CAD build for the part. Positions are in the model's coordinates, mm. Face numbers are marked on the shaded views. A direction names the side the tool comes from. Coordinates: 2 decimals unless noted, no trailing zeros. Loops run counter-clockwise (first coordinate to the right, second up) from the corner with the lowest first, then second, coordinate; pieces in that order, holes last.
1) Wall check: line 1 along Y through (x, z) = (-3.5, -20.15); line 2 along Z through (x, y) = (-1, -13.5); line 3 along Z through (x, y) = (19, -21). Give the ranges that are in metal, low to high.
2) Saw through at C-C, the plane z = -20.15. Write the cut outline in (x, y).
3) Which spindle directions (+Z, -Z, +X, -X, +Y, -Y) get a long thin tool onto all of the face, cutting with end or side? Do the marked faces 1, 2 and 3. Say none if no direction does.
4) Two-plate mould, pull along Z, no slides. Class the marked faces 4, 5 and 6: +Z half, -Z half, draft (parallel to the pull), parting line (faces both ways), or undercut.
5) Pin check, flat tips, straight feed: pin 1 Ø1.2 at (x, z) = (16, -91) entering from -Y; pin 2 Ø1 at (y, z) = (-22.5, -6) entering from +X; pin 3 Ø4 at (y, z) = (-45.5, 1.5) entering from -X; pin 4 Ø8 at (x, y) = (22.5, -15) entering from -Z (3 decimals). Stop position of each tip, or through.
6) Saw through at D-D, the plane y = -28.5. Give the number of separate pieces and of enclosed holes in the cut face, and give its area (3 significant figures).
7) Saw through at B-B, the plane y = -47.5. Write the cut outline in (x, z).
8) Saw through at A-A, the plane z = -31. Write the cut outline in (x, y).
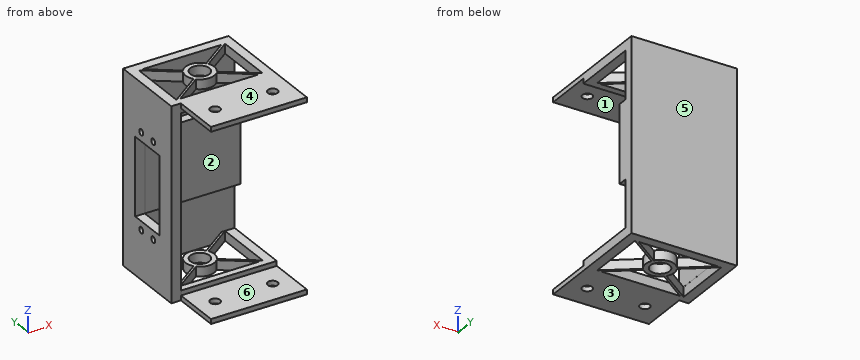
Autodesk Inventor part; units mm, degrees
ref_plane "YZ Plane" through (0, 0, 0) normal (1, 0, 0) x (0, 1, 0)
ref_plane "XZ Plane" through (0, 0, 0) normal (0, 1, 0) x (-1, 0, 0)
ref_plane "XY Plane" through (0, 0, 0) normal (0, 0, 1) x (1, 0, 0)
sketch "Esquisse1" plane through (0, 0, 0) normal (0, 0, 1) x (1, 0, 0)
  line L0 (0, 0) -> (50, 0)
  line L1 (50, 0) -> (50, -60)
  line L2 (50, -60) -> (0, -60)
  line L3 (0, -60) -> (0, 0)
  dimension "d0" = 50
  dimension "d1" = 60
extrude "Extrusion1" add sketch "Esquisse1" along normal blind 5
sketch "Esquisse2" plane through (0, 0, 0) normal (0, 0, -1) x (-1, 0, 0)
  line L0 (0, -60) -> (-50, -60)
  line L1 (-50, -60) -> (-50, -35)
  line L2 (-50, -35) -> (0, -35)
  line L3 (0, -35) -> (0, -60)
  dimension "d4" = 25
extrude "Extrusion2" cut sketch "Esquisse2" against normal blind 2.5
sketch "Esquisse4" plane through (0, 0, 2.5) normal (0, 0, -1) x (-1, 0, 0)
  circle A0 centre (-10, -47.5) radius 2.6
  circle A1 centre (-40, -47.5) radius 2.6
  line L0 (-50, -60) -> (-50, -35)
  line L1 (0, -35) -> (0, -60)
  line L2 (0, -60) -> (-50, -60)
  point P0 (0, 0)
  dimension "d7" = 10
  dimension "d8" = 10
  dimension "d9" = 5.2
  dimension "d10" = 5.2
  dimension "d11" = 12.5
  dimension "d12" = 12.5
extrude "Extrusion3" cut sketch "Esquisse4" against normal blind 2.5
sketch "Esquisse5" plane through (0, 0, 0) normal (0, 1, 0) x (1, 0, 0)
  line L0 (0, -5) -> (50, -5)
  line L1 (50, -5) -> (50, 95)
  line L2 (50, 95) -> (0, 95)
  line L3 (0, 95) -> (0, -5)
  point P0 (0, 0)
  dimension "d15" = 50
  dimension "d16" = 100
extrude "Extrusion4" add sketch "Esquisse5" along normal blind 5
sketch "Esquisse6" plane through (0, 0, 0) normal (0, -1, 0) x (1, 0, 0)
  line L0 (50, -95) -> (0, -95)
  line L1 (0, -95) -> (0, -90)
  line L2 (0, -90) -> (50, -90)
  line L3 (50, -90) -> (50, -95)
  dimension "d19" = 5
extrude "Extrusion5" add sketch "Esquisse6" along normal blind 60
sketch "Esquisse7" plane through (0, 0, -90) normal (0, 0, 1) x (1, 0, 0)
  line L0 (50, -60) -> (0, -60)
  line L1 (0, -60) -> (0, -35)
  line L2 (0, -35) -> (50, -35)
  line L3 (50, -35) -> (50, -60)
  point P0 (0, 0)
  dimension "d22" = 25
extrude "Extrusion6" cut sketch "Esquisse7" against normal blind 2.5
sketch "Esquisse8" plane through (0, 0, -92.5) normal (0, 0, 1) x (1, 0, 0)
  circle A0 centre (40, -47.5) radius 2.6
  circle A1 centre (10, -47.5) radius 2.6
  line L0 (50, -60) -> (0, -60)
  line L1 (0, -60) -> (0, -35)
  line L2 (50, -35) -> (50, -60)
  point P0 (0, 0)
  dimension "d25" = 5.2
  dimension "d26" = 5.2
  dimension "d27" = 12.5
  dimension "d28" = 12.5
  dimension "d29" = 10
  dimension "d30" = 10
extrude "Extrusion7" cut sketch "Esquisse8" against normal blind 2.5
sketch "Esquisse9" plane through (0, -60, 2.5) normal (-1, 0, 0) x (0, 0, 1)
  line L0 (2.5, 0) -> (2.5, 65)
  line L1 (2.5, 65) -> (-97.5, 65)
  line L2 (2.5, 25.0215) -> (-97.5, 25.0215)
  line L3 (-97.5, 25.0215) -> (-97.5, 65)
  line L4 (-97.5, 65) -> (2.5, 65)
  line L5 (2.5, 65) -> (2.5, 25.0215)
  point P0 (-2.5, 60)
extrude "Extrusion8" add sketch "Esquisse9" along normal blind 5
sketch "Esquisse10" plane through (-5, -60, 2.5) normal (-1, 0, 0) x (0, 0, 1)
  line L0 (-27.25, 35.0215) -> (-67.75, 35.0215)
  line L1 (-67.75, 35.0215) -> (-67.75, 55.0215)
  line L2 (-67.75, 55.0215) -> (-27.25, 55.0215)
  line L3 (-27.25, 55.0215) -> (-27.25, 35.0215)
  circle A0 centre (-22.65, 40.0215) radius 1.6
  circle A1 centre (-22.65, 50.0215) radius 1.6
  circle A2 centre (-72.35, 40.0215) radius 1.6
  circle A3 centre (-72.35, 50.0215) radius 1.6
  line L4 (2.5, 25.0215) -> (2.5, 65)
  line L5 (-97.5, 25.0215) -> (2.5, 25.0215)
  dimension "d35" = 20
  dimension "d36" = 40.5
  dimension "d37" = 3.2
  dimension "d38" = 3.2
  dimension "d39" = 3.2
  dimension "d40" = 3.2
  dimension "d41" = 10
  dimension "d42" = 5
  dimension "d43" = 4.6
  dimension "d44" = 4.6
  dimension "d45" = 5
  dimension "d46" = 5
  dimension "d47" = 4.6
  dimension "d48" = 4.6
  dimension "d49" = 29.75
  dimension "d50" = 10
extrude "Extrusion9" cut sketch "Esquisse10" against normal blind 5
sketch "Esquisse12" plane through (0, -60, 2.5) normal (1, 0, 0) x (0, 0, -1)
  line L0 (67.8734, 60) -> (27.3734, 60)
  line L1 (27.3734, 60) -> (27.3734, 55.2)
  line L2 (27.3734, 55.2) -> (67.8734, 55.2)
  line L3 (67.8734, 55.2) -> (67.8734, 60)
  point P0 (2.5, 60)
  dimension "d56" = 4.8
  dimension "d57" = 40.5
extrude "Extrusion11" add sketch "Esquisse12" along normal blind 50
sketch "Esquisse13" plane through (50, -60, -95) normal (0, 0, -1) x (-1, 0, 0)
  line L0 (55, 65) -> (55, 25.0215) construction
  line L1 (0, 65) -> (55, 65) construction
  line L2 (55, 25.0215) -> (0, 65) construction
  line L3 (0, 60) -> (0, 25) construction
  line L4 (55, 65) -> (0, 25) construction
  circle A0 centre (27.5, 45) radius 5
  circle A1 centre (27.5, 45) radius 7.5
  line L5 (50.0269, 28.6364) -> (50, 60)
  line L6 (50, 60) -> (5, 60)
  line L7 (5, 60) -> (5, 28.6364)
  line L8 (50.0269, 28.6364) -> (5, 28.6364)
  line L9 (50.0269, 28.6364) -> (33.5718, 40.5973)
  line L10 (32.8572, 39.7511) -> (48.1482, 28.6364)
  line L11 (5, 28.6364) -> (21.4385, 40.5832)
  line L12 (22.1491, 39.7448) -> (6.875, 28.6364)
  line L13 (5, 60) -> (20.8518, 48.4714)
  line L14 (6.8787, 60) -> (21.4385, 49.4168)
  line L15 (0, 60) -> (50, 60)
  line L16 (50, 60) -> (34.1482, 48.4714)
  line L17 (50, 60) -> (48.125, 60)
  line L18 (48.125, 60) -> (33.5655, 49.4113)
  dimension "d61" = 15
  dimension "d60" = 10
  dimension "d62" = 5
extrude "Extrusion12" cut sketch "Esquisse13" against normal blind 5 contours A0 | A1 L16 L5 L9 | A1 L14 L6 L18 | L10 L8 L12 A1 | A1 L11 L7 L13
sketch "Esquisse15" plane through (0, 0, 5) normal (0, 0, 1) x (1, 0, 0)
  line L0 (49.9941, 5.0518) -> (50.0216, -34.9407) construction
  line L1 (-5.0098, 4.9946) -> (49.9941, 5.0518) construction
  line L2 (50.0216, -34.9407) -> (-5.0098, 4.9946) construction
  line L3 (-5, 1.3813) -> (-5, -34.9439) construction
  line L4 (49.9941, 5.0518) -> (-5, -34.9439) construction
  circle A0 centre (22.4971, -14.9461) radius 5
  circle A1 centre (22.4971, -14.9461) radius 7.5
  line L5 (45.0151, -31.3076) -> (44.995, 0)
  line L6 (44.995, 0) -> (0, 0)
  line L7 (0, 0) -> (0, -31.3076)
  line L8 (45.0151, -31.3076) -> (0, -31.3076)
  line L9 (45.0151, -31.3076) -> (28.5574, -19.3645)
  line L10 (27.8517, -20.1975) -> (43.1363, -31.3076)
  line L11 (0, -31.3076) -> (16.4355, -19.3628)
  line L12 (17.1458, -20.2009) -> (1.8741, -31.3076)
  line L13 (0, 0) -> (15.8473, -11.4775)
  line L14 (1.8729, 0) -> (16.4172, -10.5546)
  line L15 (44.995, 0) -> (29.1456, -11.4751)
  line L16 (0, -34.9785) -> (0, 0)
  line L17 (43.0479, 0) -> (28.5626, -10.5348)
  line L18 (44.995, 0) -> (43.0479, 0)
  line L19 (0, 0) -> (50, 0)
  dimension "d73" = 15
  dimension "d72" = 10
  dimension "d74" = 5
  dimension "d77" = 0
extrude "Extrusion13" cut sketch "Esquisse15" against normal blind 10 contours A0 | A1 L15 L5 L9 | A1 L14 L6 L17 | L10 L8 L12 A1 | A1 L11 L7 L13
properties part number "Biceps2 v2" material "Plastique ABS"
Data:
1. line 1: y = -34.98 to -21.58, -18.38 to -11.58, -8.38 to 5
1. line 2: z = -95 to -65.25, -24.75 to 5
1. line 3: z = -95 to -90, 0 to 5
2. outline: (-5, -34.98) - (0, -34.98) - (0, -21.58) - (-5, -21.58) - close; (-5, -18.38) - (0, -18.38) - (0, -11.58) - (-5, -11.58) - close; (-5, -8.38) - (0, -8.38) - (0, 0) - (50, 0) - (50, 5) - (-5, 5) - close
3. face 1: +X, -X, -Y
3. face 2: +X, -Y
3. face 3: -Z, +X, -X, +Y, -Y
4. face 4: +Z half
4. face 5: draft
4. face 6: undercut
5. pin 1: stops at y = -35
5. pin 2: stops at x = 0
5. pin 3: stops at x = 0
5. pin 4: passes through
6. separate pieces: 7
6. enclosed holes: 0
6. area: 587 mm2
7. outline: (0, -95) - (7.4, -95) - (7.4, -92.5) - (0, -92.5) - close; (0, 2.5) - (7.4, 2.5) - (7.4, 5) - (0, 5) - close; (12.6, -95) - (37.4, -95) - (37.4, -92.5) - (12.6, -92.5) - close; (12.6, 2.5) - (37.4, 2.5) - (37.4, 5) - (12.6, 5) - close; (42.6, -95) - (50, -95) - (50, -92.5) - (42.6, -92.5) - close; (42.6, 2.5) - (50, 2.5) - (50, 5) - (42.6, 5) - close
8. outline: (-5, -34.98) - (0, -34.98) - (0, -24.98) - (-5, -24.98) - close; (-5, -4.98) - (0, -4.98) - (0, -4.8) - (50, -4.8) - (50, 5) - (-5, 5) - close
